from build123d import *

# Parameters (mm, degrees)
SALIENTE_EXTRUIR1_DEPTH = 7
CROQUIS2_R              = 2
CORTAR_EXTRUIR1_DEPTH   = 7.3
REDONDEO1_R             = 9.3
CHAFL_N1_SIZE           = 0.5


# Some blends are built 0.0001 mm under size
with BuildPart() as part:
    # Croquis1 → Saliente-Extruir1 (new body)
    with BuildSketch(Plane.XY):
        with BuildLine():
            Line((2.458947449, 6.3), (-2.458947449, 6.3))
            ThreePointArc((-2.458947449, 6.3), (-12.681435441, 8.663480499), (-18.6, 0))
            Line((-18.6, 0), (-25.6, 0))
            Line((-25.6, 0), (-25.6, 7.3))
            Line((-25.6, 7.3), (-18.6, 7.3))
            Line((-18.6, 7.3), (-18.6, 10.3))
            Line((-18.6, 10.3), (18.6, 10.3))
            Line((18.6, 10.3), (18.6, 7.3))
            Line((18.6, 7.3), (25.6, 7.3))
            Line((25.6, 7.3), (25.6, 0))
            Line((25.6, 0), (18.6, 0))
            ThreePointArc((18.6, 0), (12.681435441, 8.663480499), (2.458947449, 6.3))
        make_face()
    extrude(amount=SALIENTE_EXTRUIR1_DEPTH)

    # Croquis2 → Cortar-Extruir1 (cut)
    with BuildSketch(Plane(origin=(0, 7.3, 0), x_dir=(1, 0, 0), z_dir=(0, 1, 0))):
        with Locations(Location((22.1, -3.5, 0), (0, 0, 270))):
            Circle(CROQUIS2_R)
        with Locations(Location((-22.1, -3.5, 0), (0, 0, 270))):
            Circle(CROQUIS2_R)
    extrude(amount=-CORTAR_EXTRUIR1_DEPTH, mode=Mode.SUBTRACT)

    # Redondeo1
    # the kernel refuses this fillet: 9.3 mm, written as the material it takes off along each edge
    with BuildSketch(Plane(origin=(-18.6, 10.3, -17.102631376), x_dir=(0, -1, 0), z_dir=(0, 0, 1))) as redondeo1_piece_1:
        with BuildLine():
            CenterArc((9.3, 6.841052551), REDONDEO1_R, 180, 47.35769002)
            Line((0, 6.841052551), (-0.186, 6.841052551))
            Line((-0.186, 6.841052551), (-0.186, 0))
            Line((-0.186, 0), (0, -0.186))
            ThreePointArc((0, -0.186), (1.5, -0.186), (2.874, -0.136821051))
            Line((2.874, -0.136821051), (3, 0))
        make_face()
    extrude(amount=41.205262753, mode=Mode.SUBTRACT)
    with BuildSketch(Plane(origin=(18.6, 10.3, -17.102631376), x_dir=(-1, 0, 0), z_dir=(0, 0, 1))) as redondeo1_piece_2:
        with BuildLine():
            CenterArc((6.841052551, 9.3), REDONDEO1_R, 222.64230998, 47.35769002)
            Line((0, 3), (-0.136821051, 2.874))
            ThreePointArc((-0.136821051, 2.874), (-0.186, 1.5), (-0.186, 0))
            Line((-0.186, 0), (0, -0.186))
            Line((0, -0.186), (6.841052551, -0.186))
            Line((6.841052551, -0.186), (6.841052551, 0))
        make_face()
    extrude(amount=41.205262753, mode=Mode.SUBTRACT)

    # Chaflán1
    chafl_n1_edges = [part.edges().sort_by_distance(p)[0] for p in [
        (12.681435441, 8.663480499, 0),
        (0, 6.3, 0),
        (-12.681435441, 8.663480499, 0),
        (-25.6, 3.65, 0),
        (-22.1, 7.3, 0),
        (22.1, 7.3, 0),
        (25.6, 3.65, 0),
        (-22.1, 7.3, 7),
        (-25.6, 7.3, 3.5),
        (25.6, 7.3, 3.5),
        (-25.6, 3.65, 7),
        (-12.681435441, 8.663480499, 7),
        (0, 6.3, 7),
        (12.681435441, 8.663480499, 7),
        (25.6, 3.65, 7),
        (0, 10.3, 0),
        (15.493917329, 9.51704174, 0),
        (-15.493917329, 9.51704174, 0),
        (0, 10.3, 7),
        (15.493917329, 9.51704174, 7),
        (-15.493917329, 9.51704174, 7),
        (22.1, 7.3, 7),
    ]]
    chamfer(chafl_n1_edges, length=CHAFL_N1_SIZE - 0.0001)  # a hair under: the kernel refuses the full size


solid = part.part
Part model, mm, in its own coordinate system. A direction names the side the tool comes from. Coordinates: 2 decimals unless noted, no trailing zeros. Write each loop counter-clockwise with the first axis right and the second up, starting at its lowest first coordinate (ties: lowest second). Pieces come first, ordered by that corner, then holes. Notation, with made-up numbers: (3.25, -1) - (49.25, -1) arc R35 ccw to (49.25, 37) - close; hole circle Ø4 at (37, 28.5). An arc over 180 degrees is marked (long way). Put each result on its own line as item: value.
1. Band-saw the part on C-C (y = 2.75). Give the number of separate pieces and of enclosed holes in the cut face, then the cut area to 3 significant figures.
Final values:
separate pieces: 2
enclosed holes: 2
area: 77.7 mm²
2. Flat gauge pins, fed straight in: pin 1 Ø2 at (x, z) = (-20, 4.5) entering from +Y; pin 2 Ø6 at (x, y) = (-4.5, 8.5) entering from -Z; pin 3 Ø1 at (y, z) = (8.5, 4.5) entering from -X; pin 4 Ø4 at (x, z) = (13, 3) entering from -Y. Where does each tip first touch, or does it go through?
Final values:
pin 1: stops at y = 7.3
pin 2: stops at z = 0
pin 3: stops at x = -17.88
pin 4: stops at y = 7.35
3. Band-saw the part on B-B (x = 22.1). Write the cut outline in (y, z).
Final values:
outline: (0, 0) - (6.8, 0) - (7.3, 0.5) - (7.3, 1.5) - (0, 1.5) - close; (0, 5.5) - (7.3, 5.5) - (7.3, 6.5) - (6.8, 7) - (0, 7) - close
4. 3-axis set-ups, long thin cutter, end or side, ignore diameter. For faces 5 (the flat face through (-20, 7.3, 2)), 6 (the flat face through (20, 7.3, 2)), 7 (the flat face through (0, 7, 7)), 8 (the flat face through (25.6, 3, 3)), 9 (the flat face through (0, 6.3, 3)): which of +Z, -Z, +X, -X, +Y, -Y reach the whole face in a straight line?
Final values:
face 5: +Z, -Z, -X, +Y
face 6: +Z, -Z, +X, +Y
face 7: +Z, +X, -X, +Y, -Y
face 8: +Z, -Z, +X, +Y, -Y
face 9: +Z, -Z, -Y
5. Probe line 1 along X through (y, z) = (3, 3.5); line 2 along X through (y, z) = (1.75, 3.5); line 3 along Y through (x, z) = (-20.5, 6.5). List the from-to ranges inside material, lowest first. Write a range as [from, to].
Final values:
line 1: x = [-25.6, -24.1], [-20.1, -18.1], [18.1, 20.1], [24.1, 25.6]
line 2: x = [-25.6, -24.1], [-20.1, -18.43], [18.43, 20.1], [24.1, 25.6]
line 3: y = [0, 7.3]
6. Two-plate mould, pull along Z, no slides. Class faces 1 (the cylindrical face through (20.148, 3.701, 3.066)), 2 (the conical face through (15.402, 9.167, 0.142)), 3 (the cylindrical face through (15.543, 9.495, 3.458)), 4 (the conical face through (15.402, 9.167, 6.858)): +Z half, -Z half, draft (parallel to the pull), parting line (faces both ways), or undercut.
Final values:
face 1: undercut
face 2: -Z half
face 3: draft
face 4: +Z half
7. Band-saw the part on A-A (z = 3.5). Write the cut outline in (x, y), then the cut area to 3 significant figures.
Final values:
outline: (-25.6, 0) - (-24.1, 0) - (-24.1, 7.3) - (-25.1, 7.3) - (-25.6, 6.8) - close; (-20.1, 0) - (-18.6, 0) arc R9.3 cw to (-2.46, 6.3) - (2.46, 6.3) arc R9.3 cw to (18.6, 0) - (20.1, 0) - (20.1, 7.3) - (18.6, 7.3) arc R9.3 ccw to (11.76, 10.3) - (-11.76, 10.3) arc R9.3 ccw to (-18.6, 7.3) - (-20.1, 7.3) - close; (24.1, 0) - (25.6, 0) - (25.6, 6.8) - (25.1, 7.3) - (24.1, 7.3) - close
area: 133 mm²
